```python
from build123d import *

# Parameters (mm, degrees)
BOSS_EXTRUDE1_DEPTH     = 19.05
CUT_EXTRUDE1_DEPTH      = 111.168382488
CUT_EXTRUDE1_DEPTH_BACK = 111.168382488
SKETCH2_R               = 10.795
SKETCH3_W               = 76.2
SKETCH3_H               = 101.6
BOSS_EXTRUDE2_DEPTH     = 3.175


with BuildPart() as part:
    # Sketch1 → Boss-Extrude1 (new, symmetric)
    with BuildSketch(Plane.XY):
        Polygon((-38.1, 0), (38.1, 0), (38.1, 101.6), (25.4, 101.6), (25.4, 50.8), (-25.4, 50.8), (-25.4, 101.6), (-38.1, 101.6), align=None)
    extrude(amount=BOSS_EXTRUDE1_DEPTH, both=True)

    # Sketch2 → Cut-Extrude1 (cut, two sides: drawn at the far end of the back side and taken through both)
    with BuildSketch(Plane(origin=(0, 0, 0), x_dir=(0, 0, -1), z_dir=(1, 0, 0)).offset(-CUT_EXTRUDE1_DEPTH_BACK)):
        with Locations((0, 76.2)):
            Circle(SKETCH2_R)
    extrude(amount=CUT_EXTRUDE1_DEPTH + CUT_EXTRUDE1_DEPTH_BACK, mode=Mode.SUBTRACT)

    # Sketch3 → Boss-Extrude2 (add)
    with BuildSketch(Plane.XY.offset(19.05)):
        with Locations((0, 50.8)):
            Rectangle(SKETCH3_W, SKETCH3_H)
    extrude(amount=BOSS_EXTRUDE2_DEPTH)


solid = part.part
```
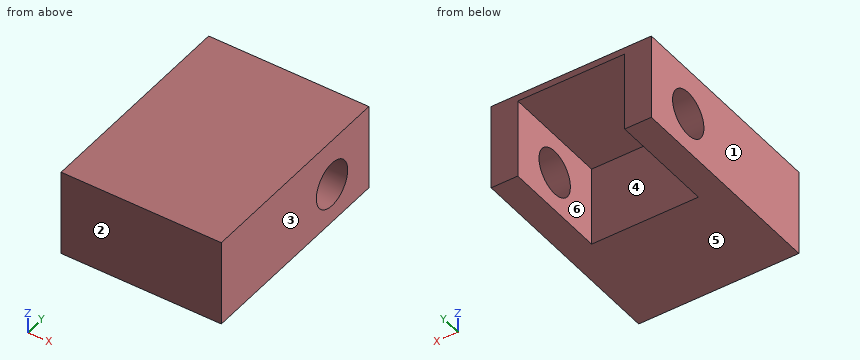
Work out the finished part from the listing and answer in its coordinate system (mm). Face numbers are marked on the shaded views. A direction names the side the tool comes from. Round coordinates to 2 decimals unless told otherwise and drop trailing zeros. Order: outer loops, then holes, each group sorted by start corner. A loop starts at its lowest first (then second) coordinate and runs counter-clockwise, first axis right, second up.
Q1. Given pin 1 Ø15 at (x, y) = (8.5, 67.5) entering from -Z; pin 2 Ø6 at (x, z) = (-21, -9) entering from +Y, each flat-ended and moving along its own axis, determine where each tip first touches the part or whether it passes through.
Solution:
pin 1: stops at z = 19.05
pin 2: stops at y = 50.8
Q2. A cutting plane is placed at A-A, the plane y = 76.2. Determine the outline of the cut face in (x, z) (3 decimals).
Solution:
outline: (-38.1, -19.05) - (-25.4, -19.05) - (-25.4, -10.795) - (-38.1, -10.795) - close; (-38.1, 10.795) - (-25.4, 10.795) - (-25.4, 19.05) - (25.4, 19.05) - (25.4, 10.795) - (38.1, 10.795) - (38.1, 22.225) - (-38.1, 22.225) - close; (25.4, -19.05) - (38.1, -19.05) - (38.1, -10.795) - (25.4, -10.795) - close
Q3. The mould has two halves that part along X. Classify the marked faces 1, 2, 3 and 4: pulls with the +X half, pulls with the -X half, needs draft (parallel to the pull), parting line crosses it, or undercut.
Solution:
face 1: pulls with the -X half
face 2: needs draft
face 3: pulls with the +X half
face 4: undercut
Q4. A cutting plane is placed at D-D, the plane y = 91.5. Determine the outline of the cut face in (x, z) (3 decimals), then the cut area to 3 significant figures.
Solution:
outline: (-38.1, -19.05) - (-25.4, -19.05) - (-25.4, 19.05) - (25.4, 19.05) - (25.4, -19.05) - (38.1, -19.05) - (38.1, 22.225) - (-38.1, 22.225) - close
area: 1,210 mm2
Q5. A cutting plane is placed at C-C, the plane x = 27. Determine the outline of the cut face in (y, z) (3 decimals).
Solution:
outline: (0, -19.05) - (101.6, -19.05) - (101.6, 22.225) - (0, 22.225) - close; hole circle Ø21.59 at (76.2, 0)
Q6. A cutting plane is placed at B-B, the plane z = 1. Determine the outline of the cut face in (x, y).
Solution:
outline: (-38.1, 0) - (38.1, 0) - (38.1, 65.45) - (25.4, 65.45) - (25.4, 50.8) - (-25.4, 50.8) - (-25.4, 65.45) - (-38.1, 65.45) - close; (-38.1, 86.95) - (-25.4, 86.95) - (-25.4, 101.6) - (-38.1, 101.6) - close; (25.4, 86.95) - (38.1, 86.95) - (38.1, 101.6) - (25.4, 101.6) - close
Q7. A tool of negligible diameter and unlimited length cuts with its end or side. For the marked faces 5 and 6, from which of +Z, -Z, +X, -X, +Y, -Y can it reach the whole face along a straight path? Write none if from no direction.
Solution:
face 5: -Z, +X, -X, +Y, -Y
face 6: -Z, +Y
Q8. Find the intervals of material crossed by line 1 along X through (y, z) = (81.5, -14.5); line 2 along Z through (x, y) = (31.5, 76.5) (3 decimals); line 3 along Y through (x, z) = (34.5, 0.5), in increasing order.
Solution:
line 1: x = -38.1 to -25.4, 25.4 to 38.1
line 2: z = -19.05 to -10.791, 10.791 to 22.225
line 3: y = 0 to 65.42, 86.98 to 101.6
